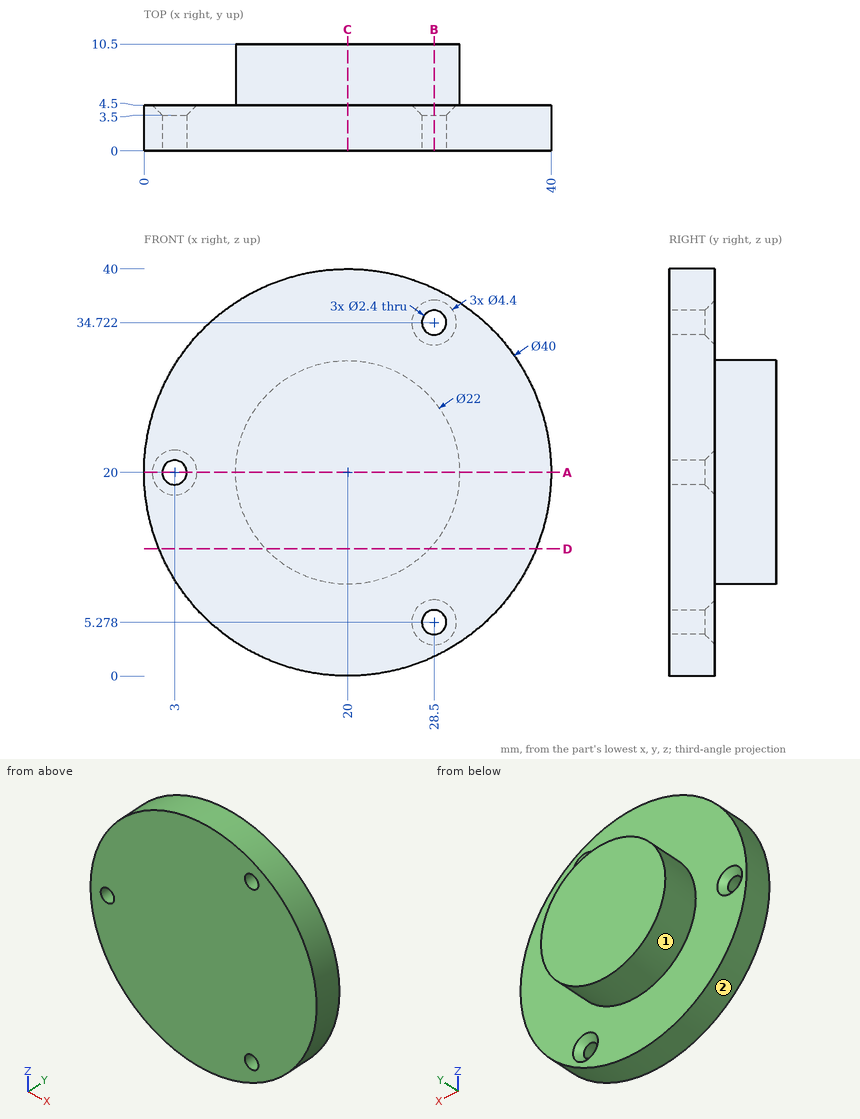
Print and shaded views of the part. All mm, measured from the part's lowest x, y and z. A direction names the side the tool comes from. Coordinates: 2 decimals unless noted, no trailing zeros. Order: outer loops, then holes, each group sorted by start corner. A loop starts at its lowest first (then second) coordinate and runs counter-clockwise, first axis right, second up. Notation, with made-up numbers: (70.25, 2.25) -> (79.25, 2.25) arc R21 cw to (79.25, 28.25) -> close; hole circle Ø5 at (-15, 73.25). An arc over 180 degrees is marked (long way). Use one line per item in the form item = value. Start each with the question number.
1) Drill centre lines: L1, parallel to Z at x = 20.5, y = 1.25; L2, parallel to Y at x = 18.5, z = 2; L3, parallel to Z at x = 28.5, y = 1.7 (1 decimal). Where is each one in solid material? Low to high. Write a range as [from, to].
2) Band-saw the part on D-D on z = 12.5. Give the cut face in (x, y).
3) Band-saw the part on A-A on z = 20. Give the cut face in (x, y).
4) Band-saw the part on C-C on x = 20. Give the cut face in (y, z), then the cut area to 3 significant figures.
5) Tool access for the marked faces 1 and 2: list every direction of +Z, -Z, +X, -X, +Y, -Y with a clear straight run to the whole face (end or side of a thin tool).
6) Drop flat-ended pins along their axis: pin 1 (3 mm diameter, centred on x = 3, z = 20, fed in from +Y); pin 2 (4 mm diameter, centred on x = 14.5, y = 3, fed in from +Z); pin 3 (5 mm diameter, centred on y = 3.5, z = 14, fed in from +X). Give the stop position or say it passes through.
7) Band-saw the part on B-B on x = 28.5. Give the cut face in (y, z).
Entries:
q1.L1 = [0.01, 39.99]
q1.L2 = [0, 4.5]
q1.L3 = [1.9, 4.1], [6.5, 33.5], [35.9, 38.1]
q2.outline = (1.46, 0) -> (38.54, 0) -> (38.54, 4.5) -> (28.05, 4.5) -> (28.05, 10.5) -> (11.95, 10.5) -> (11.95, 4.5) -> (1.46, 4.5) -> close
q3.outline = (0, 0) -> (1.8, 0) -> (1.8, 3.5) -> (0.8, 4.5) -> (0, 4.5) -> close; (4.2, 0) -> (40, 0) -> (40, 4.5) -> (31, 4.5) -> (31, 10.5) -> (9, 10.5) -> (9, 4.5) -> (5.2, 4.5) -> (4.2, 3.5) -> close
q4.outline = (0, 0) -> (4.5, 0) -> (4.5, 9) -> (10.5, 9) -> (10.5, 31) -> (4.5, 31) -> (4.5, 40) -> (0, 40) -> close
q4.area = 312 mm2
q5.face_1 = +Y
q5.face_2 = +Y, -Y
q6.pin_1 = 3.8
q6.pin_2 = 39.69
q6.pin_3 = 39.69
q7.outline = (0, 1.9) -> (4.5, 1.9) -> (4.5, 3.08) -> (3.5, 4.08) -> (0, 4.08) -> close; (0, 6.48) -> (3.5, 6.48) -> (4.5, 7.48) -> (4.5, 13.02) -> (10.5, 13.02) -> (10.5, 26.98) -> (4.5, 26.98) -> (4.5, 32.52) -> (3.5, 33.52) -> (0, 33.52) -> close; (0, 35.92) -> (3.5, 35.92) -> (4.5, 36.92) -> (4.5, 38.1) -> (0, 38.1) -> close
